```python
from build123d import *

# Parameters (mm, degrees)
BASPROSKE_W             = 12
BASPROSKE_H             = 25.5
TOOTHCUT_DEPTH          = 39.006578378
TEETHCUTS_COUNT         = 15
TEETHCUTS_ANGLE         = 336
BORSKE_R                = 0.4
BORE_DEPTH              = 50.0000508
CUT_EXTRUDE1_DEPTH      = 38.954121274
CUT_EXTRUDE1_DEPTH_BACK = 38.954121274


with BuildPart() as part:
    # BasProSke → Base-Revolve (revolve)
    with BuildSketch(Plane(origin=(0, 0, 0), x_dir=(1, 0, 0), z_dir=(0, 1, 0)), mode=Mode.PRIVATE) as base_revolve_sk:
        with Locations((6, 12.75)):
            Rectangle(BASPROSKE_W, BASPROSKE_H)
    revolve(base_revolve_sk.sketch.rotate(Axis((-10, 0, 0), (1, 0, 0)), 180), axis=Axis((-10, 0, 0), (1, 0, 0)))

    # TooCutSke → ToothCut (cut, through all)
    with BuildSketch(Plane(origin=(0, 0, 0), x_dir=(0, 0, -1), z_dir=(1, 0, 0))):
        with BuildLine():
            ThreePointArc((1.584594428, 18.681918036), (0, 18.749), (-1.584594428, 18.681918036))
            ThreePointArc((-1.584594428, 18.681918036), (-2.465052499, 22.206073835), (-4.666912141, 25.095138498))
            ThreePointArc((-4.666912141, 25.095138498), (0, 25.5254), (4.666912141, 25.095138498))
            ThreePointArc((4.666912141, 25.095138498), (2.465052499, 22.206073835), (1.584594428, 18.681918036))
        make_face()
    toothcut = extrude(amount=TOOTHCUT_DEPTH, mode=Mode.SUBTRACT)

    # TeethCuts: ToothCut ×15 about axis
    teethcuts_axis = Axis((-10, 0, 0), (1, 0, 0))
    for i in range(1, TEETHCUTS_COUNT):
        add(toothcut.rotate(teethcuts_axis, i * TEETHCUTS_ANGLE / (TEETHCUTS_COUNT - 1)), mode=Mode.SUBTRACT)

    # BorSke → Bore (cut, symmetric)
    with BuildSketch(Plane(origin=(0, 0, 0), x_dir=(0, 0, -1), z_dir=(1, 0, 0))):
        with Locations(Location((0, 0, 0), (0, 0, 180))):
            Circle(BORSKE_R)
    extrude(amount=BORE_DEPTH, both=True, mode=Mode.SUBTRACT)

    # Sketch1 → Cut-Extrude1 (cut, two sides: drawn at the far end of the back side and taken through both)
    with BuildSketch(Plane(origin=(12, 0, 0), x_dir=(0, 0, -1), z_dir=(1, 0, 0)).offset(-CUT_EXTRUDE1_DEPTH_BACK)):
        with BuildLine():
            ThreePointArc((2.5, 0), (-1.045939959, 2.270684831), (-1.624807681, -1.9))
            Line((-1.624807681, -1.9), (1.624807681, -1.9))
            ThreePointArc((1.624807681, -1.9), (2.270684831, -1.045939959), (2.5, 0))
        make_face()
    extrude(amount=CUT_EXTRUDE1_DEPTH + CUT_EXTRUDE1_DEPTH_BACK, mode=Mode.SUBTRACT)


solid = part.part
```
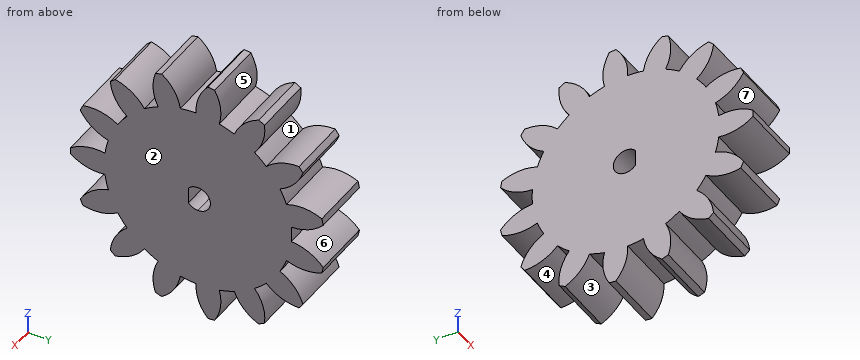
Model file for the job. Use its own axes, mm. Face numbers are marked on the shaded views. A direction names the side the tool comes from. Coordinates: 2 decimals unless noted, no trailing zeros. Write each loop counter-clockwise with the first axis right and the second up, starting at its lowest first coordinate (ties: lowest second). Pieces come first, ordered by that corner, then holes. Notation, with made-up numbers: (-1.5, -22) - (32.5, -22) arc R14 cw to (32.5, -10) - close; hole circle Ø2 at (-29.5, 37). An arc over 180 degrees is marked (long way). One line per question, with ' | ' between items. Start each with the question number.
Q1. 3-axis set-ups, long thin cutter, end or side, ignore diameter. For the marked faces 4, 5, 6 and 7: which of +Z, -Z, +X, -X, +Y, -Y reach the whole face in a straight line?
Q2. Pin check, flat tips, straight feed: pin 1 (1 mm diameter, centred on x = 5.5, z = 0.5, fed in from +Y); pin 2 (2 mm diameter, centred on x = 8.5, z = 2.5, fed in from -Y); pin 3 (1 mm diameter, centred on x = 6.5, z = 3, fed in from +Y). Stop position of each tip, or through.
Q3. Drill centre lines: line 1 (Y direction, x = 6.75, z = 19.5); line 2 (Z direction, x = 7.5, y = 2); line 3 (Y direction, x = 2.75, z = 1.5). Where is each one in solid material? Low to high. Write a range as [from, to].
Q4. Pull direction Z, two halves, no side cores. Call the marked faces 1, 2 and 3: pulls with the +Z half, pulls with the -Z half, needs draft (parallel to the pull), parting line crosses it, or undercut.
Q5. Cut at C-C, the plane y = 5.5. List the corners of the cut face in (x, z), then the cut area to 3 significant figures.
Q6. Cut at B-B, the plane z = -21. List the corners of the cut face in (x, y).
Q7. Cut at A-A, the plane z = 0. List the corners of the cut face in (x, y), then the cut area to 3 significant figures.
Q8. Cut at D-D, the plane y = -5. List the corners of the cut face in (x, z), then the cut area to 3 significant figures.
Answer below:
1) face 4: -Z, +X, -X | face 5: +X, -X | face 6: +X, -X, +Y | face 7: +X, -X, -Y
2) pin 1: y = 18.75 | pin 2: y = -24.15 | pin 3: y = 23.87
3) line 1: [-8.84, -3.76], [-0.39, 4.52], [8.48, 13.31] | line 2: [-25.42, -1.5], [1.5, 25.42] | line 3: [-24.15, -1.9], [2, 18.69]
4) face 1: undercut | face 2: needs draft | face 3: pulls with the -Z half
5) outline: (0, -17.92) - (12, -17.92) - (12, 17.92) - (0, 17.92) - close | area: 430 mm^2
6) outline: (0, -8.99) - (12, -8.99) - (12, -4.32) - (0, -4.32) - close; (0, -0.24) - (12, -0.24) - (12, 4.59) - (0, 4.59) - close; (0, 9.89) - (12, 9.89) - (12, 13.38) - (0, 13.38) - close
7) outline: (0, -25.5) - (12, -25.5) - (12, -1.9) - (0, -1.9) - close; (0, 2.5) - (12, 2.5) - (12, 18.75) - (0, 18.75) - close | area: 478 mm^2
8) outline: (0, -22.18) - (12, -22.18) - (12, 22.18) - (0, 22.18) - close | area: 532 mm^2
